Here's how the part is built. I have some questions about the finished solid (model axes, mm). A direction names the side the tool comes from. Give positions to 0.01 mm unless a question says otherwise; leave off trailing zeros. Loops run counter-clockwise (first coordinate to the right, second up) from the corner with the lowest first, then second, coordinate; pieces in that order, holes last. Notation, with made-up numbers: M 55,15.5 L 92,15.5 A27 cw 92,47.5 Z; hole C 87,59.5 d6. An arc over 180 degrees is marked long. Answer as CSV lines item,"result". Start each with the question number.
Item 1: Will this pin go through, and if not, where does the flat tip stop? P1, Ø1, axis at y = 6.5, z = 7.5, coming from the -X side.
Item 2: I want a section at D-D on y = 10.5. List the corners of the cut face in (x, z) for me.
Item 3: If I drill on line 1 along Y through (x, z) = (30, 6.5); line 2 along X through (y, z) = (25, 33); line 3 along X through (y, z) = (11, 45.5), over which ranges is the centre line in solid material (lowest first)? Write a range as from..to.
Item 4: I want a section at C-C on z = 25.5. List the corners of the cut face in (x, y) for me, plus the area to 3 significant figures.
Item 5: I want a section at B-B on x = 2.5. List the corners of the cut face in (y, z) for me.
Item 6: I want a section at A-A on y = 3.5. List the corners of the cut face in (x, z) for me.
Item 7: If we mould it in two halves opening along X, with no side actions, what happens to faces 4 (the flat face through (10, 21.1, 25)), 5 (the flat face through (5, -4, 20)), 6 (the flat face through (-6, 11, 0))? For each: released by +X, released by -X, zero draft, split by the parting line, or undercut.
Item 8: For faces 1 (the flat face through (0, 10, 25)), 2 (the flat face through (5, 25, 20)), 3 (the cylindrical face through (25.43, 23.83, 16.03)), which set-ups out of +Z, -Z, +X, -X, +Y, -Y let a thin tool reach every point of the face, with its end or its side?
from build123d import *

# Parameters (mm, degrees)
SKETCH_1_W               = 45.1
SKETCH_1_H               = 39.1
SKETCH_1_W_2             = 21.1
SKETCH_1_H_2             = 21.1
EXTRUDE_1_DEPTH          = 50
SKETCH_2_W               = 12
SKETCH_2_H               = 4.2
CUT_EXTRUDE_1_DEPTH      = 10
CUT_EXTRUDE_2_DEPTH      = 30
CUT_EXTRUDE_2_DEPTH_BACK = 30
SKETCH_3_R               = 2.1
SKETCH_4_W               = 12
SKETCH_4_H               = 4.2
CUT_EXTRUDE_3_DEPTH      = 10
CUT_EXTRUDE_4_DEPTH      = 30
CUT_EXTRUDE_4_DEPTH_BACK = 30
SKETCH_5_R               = 2.1
SKETCH_6_W               = 4.2
SKETCH_6_H               = 10.2
CUT_EXTRUDE_5_DEPTH      = 80
CUT_EXTRUDE_6_DEPTH      = 80
CUT_EXTRUDE_6_DEPTH_BACK = 80
SKETCH_7_R               = 2.1
FILLET_1_R               = 1


with BuildPart() as part:
    # 草图1 → 凸台-拉伸1 (new body)
    with BuildSketch(Plane.XY):
        with Locations((10.55, 10.55)):
            Rectangle(SKETCH_1_W, SKETCH_1_H)
        with Locations((10.55, 10.55)):
            Rectangle(SKETCH_1_W_2, SKETCH_1_H_2, mode=Mode.SUBTRACT)
    extrude(amount=EXTRUDE_1_DEPTH)

    # 草图2 → 切除-拉伸1 (cut)
    with BuildSketch(Plane.XY.offset(50)):
        with Locations((27.1, 14.65)):
            Rectangle(SKETCH_2_W, SKETCH_2_H)
        with Locations((27.1, 6.45)):
            Rectangle(SKETCH_2_W, SKETCH_2_H)
        with Locations((-6, 6.45)):
            Rectangle(SKETCH_2_W, SKETCH_2_H)
        with Locations((-6, 14.65)):
            Rectangle(SKETCH_2_W, SKETCH_2_H)
    extrude(amount=-CUT_EXTRUDE_1_DEPTH, mode=Mode.SUBTRACT)

    # 草图3 → 切除-拉伸2 (cut, two sides: drawn at the far end of the back side and taken through both)
    with BuildSketch(Plane(origin=(0, 12.55, 0), x_dir=(1, 0, 0), z_dir=(0, 1, 0)).offset(-CUT_EXTRUDE_2_DEPTH_BACK)):
        with Locations(Location((25.6, -45.5, 0), (0, 0, 90))):
            Circle(SKETCH_3_R)
        with Locations(Location((-4.5, -45.5, 0), (0, 0, 90))):
            Circle(SKETCH_3_R)
    extrude(amount=CUT_EXTRUDE_2_DEPTH + CUT_EXTRUDE_2_DEPTH_BACK, mode=Mode.SUBTRACT)

    # 草图4 → 切除-拉伸3 (cut)
    with BuildSketch(Plane(origin=(0, 0, 0), x_dir=(-1, 0, 0), z_dir=(0, 0, -1))):
        with Locations((6, 6.45)):
            Rectangle(SKETCH_4_W, SKETCH_4_H)
        with Locations((6, 14.65)):
            Rectangle(SKETCH_4_W, SKETCH_4_H)
        with Locations((-27.1, 6.45)):
            Rectangle(SKETCH_4_W, SKETCH_4_H)
        with Locations((-27.1, 14.65)):
            Rectangle(SKETCH_4_W, SKETCH_4_H)
    extrude(amount=-CUT_EXTRUDE_3_DEPTH, mode=Mode.SUBTRACT)

    # 草图5 → 切除-拉伸4 (cut, two sides: drawn at the far end of the back side and taken through both)
    with BuildSketch(Plane(origin=(0, 12.55, 0), x_dir=(1, 0, 0), z_dir=(0, 1, 0)).offset(-CUT_EXTRUDE_4_DEPTH_BACK)):
        with Locations(Location((25.6, -4.5, 0), (0, 0, 90))):
            Circle(SKETCH_5_R)
        with Locations(Location((-4.5, -4.5, 0), (0, 0, 90))):
            Circle(SKETCH_5_R)
    extrude(amount=CUT_EXTRUDE_4_DEPTH + CUT_EXTRUDE_4_DEPTH_BACK, mode=Mode.SUBTRACT)

    # 草图6 → 切除-拉伸5 (cut)
    with BuildSketch(Plane(origin=(0, 30.1, 0), x_dir=(1, 0, 0), z_dir=(0, 1, 0))):
        with Locations((15.868916464, -14.9)):
            Rectangle(SKETCH_6_W, SKETCH_6_H)
        with Locations((5.231083536, -14.9)):
            Rectangle(SKETCH_6_W, SKETCH_6_H)
        with Locations((5.231083536, -35.1)):
            Rectangle(SKETCH_6_W, SKETCH_6_H)
        with Locations((15.868916464, -35.1)):
            Rectangle(SKETCH_6_W, SKETCH_6_H)
    extrude(amount=-CUT_EXTRUDE_5_DEPTH, mode=Mode.SUBTRACT)

    # 草图7 → 切除-拉伸6 (cut, two sides: drawn at the far end of the back side and taken through both)
    with BuildSketch(Plane(origin=(13.768916464, 0, 0), x_dir=(0, 0, -1), z_dir=(1, 0, 0)).offset(-CUT_EXTRUDE_6_DEPTH_BACK)):
        with Locations(Location((-35.1, 25.6, 0), (0, 0, 180))):
            Circle(SKETCH_7_R)
        with Locations(Location((-14.9, 25.6, 0), (0, 0, 180))):
            Circle(SKETCH_7_R)
        with Locations(Location((-14.9, -4.5, 0), (0, 0, 180))):
            Circle(SKETCH_7_R)
        with Locations(Location((-35.1, -4.5, 0), (0, 0, 180))):
            Circle(SKETCH_7_R)
    extrude(amount=CUT_EXTRUDE_6_DEPTH + CUT_EXTRUDE_6_DEPTH_BACK, mode=Mode.SUBTRACT)

    # 圆角1
    fillet_1_edges = [part.edges().sort_by_distance(p)[0] for p in [
        (21.1, 10.55, 0),
        (0, 10.55, 0),
        (33.1, 10.55, 0),
        (33.1, 23.425, 0),
        (-12, 10.55, 0),
        (-12, -2.325, 0),
        (33.1, -2.325, 50),
        (0, 14.65, 10),
        (-12, 14.65, 10),
        (21.1, 6.45, 10),
        (33.1, 6.45, 10),
        (21.1, 14.65, 10),
        (33.1, 14.65, 10),
        (0, 6.45, 10),
        (-12, 6.45, 10),
        (10.55, 30.1, 50),
        (15.868916464, -9, 30),
        (15.868916464, -9, 40.2),
        (15.868916464, 30.1, 40.2),
        (15.868916464, 30.1, 30),
        (5.231083536, -9, 40.2),
        (5.231083536, -9, 30),
        (5.231083536, 30.1, 40.2),
        (5.231083536, 30.1, 30),
        (5.231083536, -9, 20),
        (5.231083536, -9, 9.8),
        (5.231083536, 30.1, 9.8),
        (5.231083536, 30.1, 20),
        (15.868916464, -9, 9.8),
        (15.868916464, -9, 20),
        (15.868916464, 30.1, 20),
        (15.868916464, 30.1, 9.8),
        (21.1, 10.55, 50),
        (0, 10.55, 50),
        (33.1, 10.55, 50),
        (33.1, 23.425, 50),
        (-12, 10.55, 50),
        (-12, -2.325, 50),
        (0, 14.65, 40),
        (-12, 14.65, 40),
        (-12, 23.425, 50),
        (10.55, 30.1, 0),
        (33.1, -2.325, 0),
        (0, 6.45, 40),
        (-12, 6.45, 40),
        (10.55, -9, 0),
        (21.1, 6.45, 40),
        (33.1, 6.45, 40),
        (-12, 23.425, 0),
        (21.1, 14.65, 40),
        (33.1, 14.65, 40),
        (-12, 30.1, 25),
        (33.1, 30.1, 25),
        (33.1, -9, 25),
        (-12, -9, 25),
        (10.55, -9, 50),
    ]]
    fillet(fillet_1_edges, radius=FILLET_1_R)


solid = part.part
Result:
1,P1,"through"
2,outline,"M -12,1 A1 ccw -11,0 L -1,0 A1 ccw 0,1 L 0,49 A1 ccw -1,50 L -11,50 A1 ccw -12,49 Z; M 21.1,1 A1 ccw 22.1,0 L 32.1,0 A1 ccw 33.1,1 L 33.1,49 A1 ccw 32.1,50 L 22.1,50 A1 ccw 21.1,49 Z; hole C -4.5,4.5 d4.2; hole C -4.5,45.5 d4.2; hole C 25.6,4.5 d4.2; hole C 25.6,45.5 d4.2"
3,line 1,"-9..4.35, 8.55..12.55, 16.75..30.1"
3,line 2,"-12..3.13, 7.33..13.77, 17.97..33.1"
3,line 3,"-12..-6.6, -2.4..0, 21.1..23.5, 27.7..33.1"
4,outline,"M -12,-8 A1 ccw -11,-9 L 32.1,-9 A1 ccw 33.1,-8 L 33.1,29.1 A1 ccw 32.1,30.1 L -11,30.1 A1 ccw -12,29.1 Z; hole M 0,0 L 21.1,0 L 21.1,21.1 L 0,21.1 Z"
4,area,"1,320 mm^2"
5,outline,"M -9,1 A1 ccw -8,0 L 0,0 L 0,50 L -8,50 A1 ccw -9,49 Z; M 21.1,0 L 29.1,0 A1 ccw 30.1,1 L 30.1,49 A1 ccw 29.1,50 L 21.1,50 Z; hole C -4.5,14.9 d4.2; hole C -4.5,35.1 d4.2; hole C 25.6,14.9 d4.2; hole C 25.6,35.1 d4.2"
6,outline,"M -12,1 A1 ccw -11,0 L 0,0 L 0,50 L -11,50 A1 ccw -12,49 Z; M 21.1,0 L 32.1,0 A1 ccw 33.1,1 L 33.1,49 A1 ccw 32.1,50 L 21.1,50 Z; hole C -4.5,4.5 d4.2; hole C -4.5,45.5 d4.2; hole C 25.6,4.5 d4.2; hole C 25.6,45.5 d4.2"
7,face 4,"undercut"
7,face 5,"undercut"
7,face 6,"zero draft"
8,face 1,"+Z, -Z"
8,face 2,"+Y, -Y"
8,face 3,"+X, -X"
